Print and shaded views of the part. All mm, measured from the part's lowest x, y and z. A direction names the side the tool comes from. Round coordinates to 2 decimals unless told otherwise and drop trailing zeros. Write each loop counter-clockwise with the first axis right and the second up, starting at its lowest first coordinate (ties: lowest second). Pieces come first, ordered by that corner, then holes. Notation, with made-up numbers: (52.25, 77) - (76.25, 77) arc R26 cw to (76.25, 95) - close; hole circle Ø8 at (-9.5, 66.25). An arc over 180 degrees is marked (long way). One line per item, written item: value.
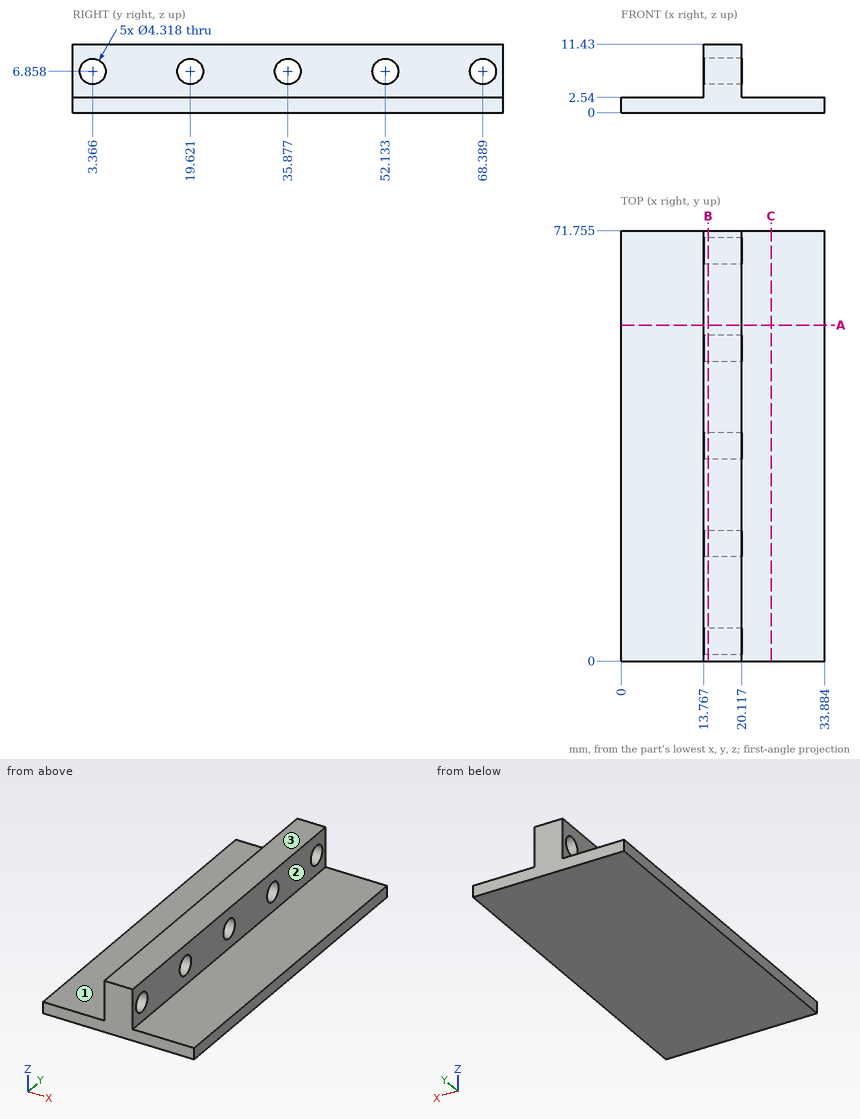
1. Band-saw the part on C-C on x = 25. Write the cut outline in (y, z) (1 decimal).
Report:
outline: (0, 0) - (71.8, 0) - (71.8, 2.5) - (0, 2.5) - close
2. Wall check: probe 1 along Y at (x, z) = (15.5, 5) (1 decimal); probe 2 along Z at (x, y) = (4, 42); probe 3 along X at (y, z) = (10, 10.5). Give the ranges that are in metal, low to high. Write a range as [from, to].
Report:
probe 1: [0, 2.3], [4.5, 18.5], [20.7, 34.8], [37, 51], [53.2, 67.3], [69.5, 71.8]
probe 2: [0, 2.54]
probe 3: [13.77, 20.12]
3. Band-saw the part on A-A on y = 56. Write the cut outline in (x, z).
Report:
outline: (0, 0) - (33.88, 0) - (33.88, 2.54) - (20.12, 2.54) - (20.12, 11.43) - (13.77, 11.43) - (13.77, 2.54) - (0, 2.54) - close
4. Drop flat-ended pins along their axis: pin 1 (6 mm diameter, centred on y = 15.5, z = 8.5, fed in from -X); pin 2 (5 mm diameter, centred on y = 35.88, z = 6.86, fed in from +X); pin 3 (2 mm diameter, centred on x = 9.5, z = 4, fed in from +Y); pin 4 (15 mm diameter, centred on x = 3.5, y = 48, fed in from +Z). Give the stop position or say it passes through.
Report:
pin 1: x = 13.77
pin 2: x = 20.12
pin 3: through
pin 4: z = 2.54
5. Band-saw the part on B-B on x = 14.5. Write the cut outline in (y, z) (1 decimal), plus the area to 3 significant figures.
Report:
outline: (0, 0) - (71.8, 0) - (71.8, 11.4) - (0, 11.4) - close; hole circle Ø4.3 at (3.4, 6.9); hole circle Ø4.3 at (19.6, 6.9); hole circle Ø4.3 at (35.9, 6.9); hole circle Ø4.3 at (52.1, 6.9); hole circle Ø4.3 at (68.4, 6.9)
area: 747 mm²
6. Tool access for the marked faces 1, 2 and 3: list every direction of +Z, -Z, +X, -X, +Y, -Y with a clear straight run to the whole face (end or side of a thin tool).
Report:
face 1: +Z, -X, +Y, -Y
face 2: +Z, +X, +Y, -Y
face 3: +Z, +X, -X, +Y, -Y
